Source: CAD feature listing. Evaluate the final solid. Frame: model axes, mm. A direction names the side the tool comes from. Coordinates: 2 decimals unless noted, no trailing zeros. Order: outer loops, then holes, each group sorted by start corner. A loop starts at its lowest first (then second) coordinate and runs counter-clockwise, first axis right, second up. Notation, with made-up numbers: (61.25, 67) -> (80.25, 67) arc R18 cw to (80.25, 82) -> close; hole circle Ø6 at (2.25, -16). An arc over 180 degrees is marked (long way). Put each result on its own line as item: value.
from build123d import *

# Parameters (mm, degrees)
SKETCH_1_R             = 2.8
EXTRUDE_1_DEPTH        = 26
SKETCH_2_R             = 1.65
CUT_EXTRUDE_2_DEPTH    = 43.555295324
CUT_EXTRUDE_2120_REACH = 46.4
SKETCH_4_W             = 26
SKETCH_4_H             = 3
CUT_EXTRUDE_3_REACH    = 44.395
SKETCH_7_W             = 26
SKETCH_7_H             = 3


with BuildPart() as part:
    # 草图1 → 凸台-拉伸1 (new body)
    with BuildSketch(Plane.XY):
        with BuildLine():
            Line((3, 6), (3, 24.5))
            Line((3, 24.5), (7.8, 24.5))
            Line((7.8, 24.5), (7.8, 30.5))
            Line((7.8, 30.5), (0, 30.5))
            Line((0, 30.5), (-10.13168569, 18.471060485))
            ThreePointArc((-10.13168569, 18.471060485), (-11.307451211, 15.25), (-10.13168569, 12.028939515))
            Line((-10.13168569, 12.028939515), (0, 0))
            Line((0, 0), (7.8, 0))
            Line((7.8, 0), (7.8, 6))
            Line((7.8, 6), (3, 6))
        make_face()
        with Locations(Location((-5, 15.25, 0), (0, 0, 180))):
            Circle(SKETCH_1_R, mode=Mode.SUBTRACT)
    extrude(amount=EXTRUDE_1_DEPTH)

    # 草图2 → 切除-拉伸2 (cut, through all)
    with BuildSketch(Plane(origin=(3, 0, 0), x_dir=(0, 0, -1), z_dir=(1, 0, 0))):
        with Locations((-3.5, 20.75)):
            Circle(SKETCH_2_R)
        with Locations((-22.5, 9.75)):
            Circle(SKETCH_2_R)
        with Locations((-22.5, 20.75)):
            Circle(SKETCH_2_R)
        with Locations((-3.5, 9.75)):
            Circle(SKETCH_2_R)
    extrude(amount=-CUT_EXTRUDE_2_DEPTH, mode=Mode.SUBTRACT)

    # 草图4 → Cut-Extrude 2120 (cut, up to next)
    with BuildSketch(Plane(origin=(7.8, 0, 0), x_dir=(0, 0, -1), z_dir=(1, 0, 0)), mode=Mode.PRIVATE) as cut_extrude_2120_sk1:
        with Locations((-13, 29)):
            Rectangle(SKETCH_4_W, SKETCH_4_H)
    cut_extrude_2120_tool1 = extrude(cut_extrude_2120_sk1.sketch, amount=-CUT_EXTRUDE_2120_REACH, mode=Mode.PRIVATE) & part.part
    # 草图4 → Cut-Extrude 2120 (cut, up to next)
    with BuildSketch(Plane(origin=(7.8, 0, 0), x_dir=(0, 0, -1), z_dir=(1, 0, 0)), mode=Mode.PRIVATE) as cut_extrude_2120_sk2:
        with Locations((-13, 1.5)):
            Rectangle(SKETCH_4_W, SKETCH_4_H)
    cut_extrude_2120_tool2 = extrude(cut_extrude_2120_sk2.sketch, amount=-CUT_EXTRUDE_2120_REACH, mode=Mode.PRIVATE) & part.part
    add(cut_extrude_2120_tool1.solids().sort_by_distance((7.8, 29, 13))[0], mode=Mode.SUBTRACT)
    add(cut_extrude_2120_tool2.solids().sort_by_distance((7.8, 1.5, 13))[0], mode=Mode.SUBTRACT)

    # 切除-拉伸3: up to this plane
    cut_extrude_3_end = Plane(origin=(0, 0, 26), z_dir=(0.7648468958435873, 0.6442120969978977, 0))
    # 草图7 → 切除-拉伸3 (cut, up to the surface)
    with BuildSketch(Plane(origin=(7.8, 0, 0), x_dir=(0, 0, -1), z_dir=(1, 0, 0)), mode=Mode.PRIVATE) as cut_extrude_3_sk1:
        with Locations((-13, 4.5)):
            Rectangle(SKETCH_7_W, SKETCH_7_H)
    cut_extrude_3_tool1 = split(extrude(cut_extrude_3_sk1.sketch, amount=-CUT_EXTRUDE_3_REACH, mode=Mode.PRIVATE), bisect_by=cut_extrude_3_end, keep=Keep.BOTH, mode=Mode.PRIVATE)
    add(cut_extrude_3_tool1.solids().sort_by_distance((7.8, 4.5, 13))[0], mode=Mode.SUBTRACT)


solid = part.part
1. Cut plane B-B on y = 15.25. Output: boundary loops of the cut face in (x, z).
Numbers:
outline: (-11.31, 0) -> (-7.8, 0) -> (-7.8, 26) -> (-11.31, 26) -> close; (-2.2, 0) -> (3, 0) -> (3, 26) -> (-2.2, 26) -> close
2. Cut plane A-A on z = 13. Output: boundary loops of the cut face in (x, y).
Numbers:
outline: (-10.13, 12.03) -> (-5.05, 6) -> (3, 6) -> (3, 24.5) -> (7.8, 24.5) -> (7.8, 27.5) -> (-2.53, 27.5) -> (-10.13, 18.47) arc R5 ccw to start; hole circle Ø5.6 at (-5, 15.25)
3. Ray query, line 1 along Y through (x, z) = (0, 3.5); line 2 along Z through (x, y) = (-0.25, 9.75); line 3 along Y through (x, z) = (-2.5, 24). Return the intervals inside material, ascending.
Numbers:
line 1: y = 6 to 8.1, 11.4 to 19.1, 22.4 to 27.5
line 2: z = 0 to 1.85, 5.15 to 20.85, 24.15 to 26
line 3: y = 6 to 9.06, 10.44 to 13.99, 16.51 to 20.06, 21.44 to 27.5
4. Pull-direction query (Z, two-part tool) for faces 3 (the cylindrical face through (-3.213, 11.386, 22.715)), 4 (the flat face through (-2, 17, 0)), 5 (the flat face through (3, 15, 13)); classes: pulls with the +Z half, pulls with the -Z half, needs draft (parallel to the pull), parting line crosses it, or undercut.
Numbers:
face 3: undercut
face 4: pulls with the -Z half
face 5: needs draft
5. Set-up query: faces 1 (the flat face through (-1, 6, 13)), 2 (the flat face through (5, 24.5, 13)). Return all of +Z, -Z, +X, -X, +Y, -Y with unobstructed straight access to the full face (end or side cutting, diameter ignored); none if empty.
Numbers:
face 1: +Z, -Z, +X, -X, -Y
face 2: +Z, -Z, +X, -Y
6. Cut plane C-C on x = -5.5. Output: boundary loops of the cut face in (y, z) (3 decimals).
Numbers:
outline: (6.53, 0) -> (12.495, 0) -> (12.495, 26) -> (6.53, 26) -> close; (18.005, 0) -> (23.97, 0) -> (23.97, 26) -> (18.005, 26) -> close; hole circle Ø3.3 at (9.75, 3.5); hole circle Ø3.3 at (9.75, 22.5); hole circle Ø3.3 at (20.75, 3.5); hole circle Ø3.3 at (20.75, 22.5)
7. Cut plane D-D on z = 22.5. Output: boundary loops of the cut face in (x, y), plus the area to 3 significant figures.
Numbers:
outline: (-10.13, 12.03) -> (-9.6, 11.4) -> (3, 11.4) -> (3, 19.1) -> (-9.6, 19.1) -> (-10.13, 18.47) arc R5 ccw to start; (-6.82, 8.1) -> (-5.05, 6) -> (3, 6) -> (3, 8.1) -> close; (-6.82, 22.4) -> (3, 22.4) -> (3, 24.5) -> (7.8, 24.5) -> (7.8, 27.5) -> (-2.53, 27.5) -> close; hole circle Ø5.6 at (-5, 15.25)
area: 154 mm2
8. First-contact query: pin 1 (2.5 mm diameter, centred on y = 20.75, z = 22.5, fed in from +X); pin 2 (4.5 mm diameter, centred on y = 9.75, z = 22.5, fed in from +X); pin 3 (5 mm diameter, centred on y = 20.5, z = 19.5, fed in from -X); pin 4 (1.4 mm diameter, centred on x = 5.5, z = 7.5, fed in from -Y). Flat tips, straight axial feed; report the tip coordinate or a pass-through.
Numbers:
pin 1: passes through
pin 2: stops at x = 3
pin 3: stops at x = -10.48
pin 4: stops at y = 24.5
